from build123d import *

# Parameters (mm, degrees)
SKETCH1_R           = 2.75
BOSS_EXTRUDE1_DEPTH = 100
SKETCH3_W           = 4
SKETCH3_H           = 3.5
BOSS_EXTRUDE2_DEPTH = 10
SKETCH4_W           = 4
SKETCH4_H           = 3.5
BOSS_EXTRUDE3_DEPTH = 10


with BuildPart() as part:
    # Sketch1 → Boss-Extrude1 (new body)
    with BuildSketch(Plane.XY):
        Circle(SKETCH1_R)
    extrude(amount=BOSS_EXTRUDE1_DEPTH)

    # Sketch3 → Boss-Extrude2 (add)
    with BuildSketch(Plane.XY.offset(100)):
        Rectangle(SKETCH3_W, SKETCH3_H)
    extrude(amount=BOSS_EXTRUDE2_DEPTH)

    # Sketch4 → Boss-Extrude3 (add)
    with BuildSketch(Plane(origin=(0, 0, 0), x_dir=(-1, 0, 0), z_dir=(0, 0, -1))):
        Rectangle(SKETCH4_W, SKETCH4_H)
    extrude(amount=BOSS_EXTRUDE3_DEPTH)


solid = part.part
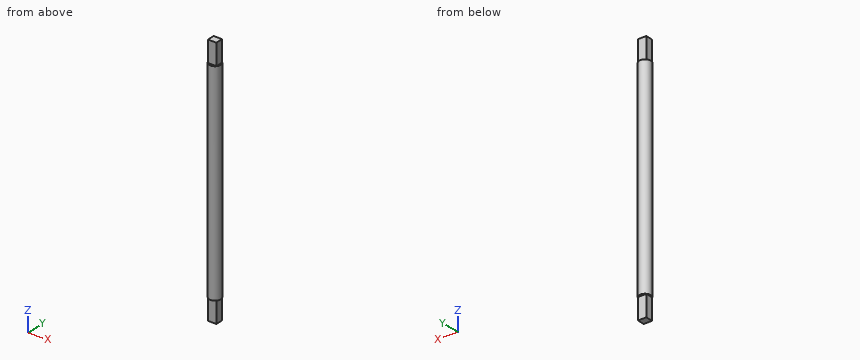
Design review of the part built by this model. Coordinates are the model's own, in mm. Give positions to 0.01 mm unless a question says otherwise; leave off trailing zeros. Order: outer loops, then holes, each group sorted by start corner. A loop starts at its lowest first (then second) coordinate and runs counter-clockwise, first axis right, second up. Notation, with made-up numbers: (-13, 40) - (10, 40) arc R21 cw to (10, 51) - close; hole circle Ø11 at (3.5, 86). An arc over 180 degrees is marked (long way). Use CSV: the item, a comma, the result in double quotes. Start each with the question number.
Q1. Take a section at C-C (z = 40). State the section outline as (x, y) points.
Q2. Take a section at A-A (x = 0). State the section outline as (y, z) points.
Q3. Take a section at B-B (y = 0). State the section outline as (x, z) points.
Q4. For P1, Ø3, axis at x = -1, z = 107, coming from the -Y side; P2, Ø2, axis at x = -0.5, z = 104.5, coming from the +Y side; P3, Ø1, axis at y = 0.5, z = -7, coming from the -X side, all flat-tipped, find the tip position at first contact; note any pin that passes through.
Q5. For line 1 (Y direction, x = 0.25, z = 12); line 2 (X direction, y = -0.1, z = 72); line 3 (Z direction, x = 2.2, y = -0.25), list the stretches that pass through material, from the lowest coordinate up.
Calculated:
1,outline,"circle Ø5.5 at (0, 0)"
2,outline,"(-2.75, 0) - (-1.75, 0) - (-1.75, -10) - (1.75, -10) - (1.75, 0) - (2.75, 0) - (2.75, 100) - (1.75, 100) - (1.75, 110) - (-1.75, 110) - (-1.75, 100) - (-2.75, 100) - close"
3,outline,"(-2.75, 0) - (-2, 0) - (-2, -10) - (2, -10) - (2, 0) - (2.75, 0) - (2.75, 100) - (2, 100) - (2, 110) - (-2, 110) - (-2, 100) - (-2.75, 100) - close"
4,P1,"stops at y = -1.75"
4,P2,"stops at y = 1.75"
4,P3,"stops at x = -2"
5,line 1,"y = -2.74 to 2.74"
5,line 2,"x = -2.75 to 2.75"
5,line 3,"z = 0 to 100"
